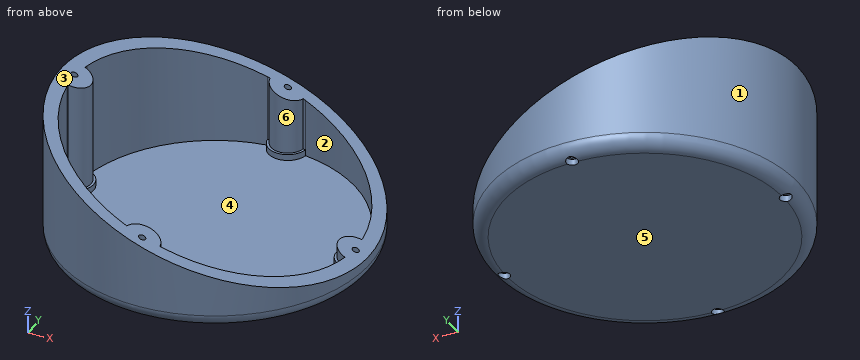
from build123d import *

# Parameters (mm, degrees)
SKETCH_1_R                = 57
EXTRUDE_1_DEPTH           = 50
CUT_EXTRUDE_1_DEPTH       = 95.857788294
CUT_EXTRUDE_1_DEPTH_BACK  = 95.857788294
FILLET_1_R                = 5
HOLE_WIZARD_1_D           = 2.4
HOLE_WIZARD_1_CBORE_D     = 4.3
HOLE_WIZARD_1_CBORE_DEPTH = 2.3
PATTERN_CIRCULAR_1_COUNT  = 4
SHELL_START               = 5
SHELL_1_DEPTH             = 43.047767655
SHELL_START_2             = 7.3
SHELL_1_2_DEPTH           = 40.747767655


# Read off the part's stored shape, not the designer's step: 抽壳1
with BuildPart() as part:
    # 草图1 → 凸台-拉伸1 (new body)
    with BuildSketch(Plane.XY):
        Circle(SKETCH_1_R)
    extrude(amount=EXTRUDE_1_DEPTH)

    # 草图2 → 切除-拉伸1 (cut, two sides: drawn at the far end of the back side and taken through both)
    with BuildSketch(Plane(origin=(0, 0, 0), x_dir=(1, 0, 0), z_dir=(0, 1, 0)).offset(-CUT_EXTRUDE_1_DEPTH_BACK)):
        Polygon((-57, -50), (57, -50), (57, -8.507393294), align=None)
    extrude(amount=CUT_EXTRUDE_1_DEPTH + CUT_EXTRUDE_1_DEPTH_BACK, mode=Mode.SUBTRACT)

    # 圆角1
    fillet_1_edges = [part.edges().sort_by_distance(p)[0] for p in [
        (-57, 0, 0),
    ]]
    fillet(fillet_1_edges, radius=FILLET_1_R)

    # 打孔尺寸(%根据)内六角圆柱头螺钉的类型1 (through all)
    with Locations(Plane(origin=(0, 0, 0), x_dir=(-1, 0, 0), z_dir=(0, 0, -1))):
        with Locations((0, 52.5)):
            hole_wizard_1 = CounterBoreHole(HOLE_WIZARD_1_D / 2, HOLE_WIZARD_1_CBORE_D / 2, HOLE_WIZARD_1_CBORE_DEPTH)

    # 阵列(圆周)1: 打孔尺寸(%根据)内六角圆柱头螺钉的类型1 ×4 about axis
    pattern_circular_1_axis = Axis((0, 0, 0), (0, 0, 1))
    for i in range(1, PATTERN_CIRCULAR_1_COUNT):
        add(hole_wizard_1.rotate(pattern_circular_1_axis, i * 360 / PATTERN_CIRCULAR_1_COUNT), mode=Mode.SUBTRACT)

    # 抽壳1 outline → 抽壳1 (cut)
    with BuildSketch(Plane.XY.offset(SHELL_START)):
        with BuildLine():
            ThreePointArc((7.081896621, -51.5155), (36.769552622, -36.769552622), (51.5155, -7.081896621))
            ThreePointArc((51.5155, -7.081896621), (45.35, 0), (51.5155, 7.081896621))
            ThreePointArc((51.5155, 7.081896621), (36.769552622, 36.769552622), (7.081896621, 51.5155))
            ThreePointArc((7.081896621, 51.5155), (0, 45.35), (-7.081896621, 51.5155))
            ThreePointArc((-7.081896621, 51.5155), (-36.769552622, 36.769552622), (-51.5155, 7.081896621))
            ThreePointArc((-51.5155, 7.081896621), (-45.35, 0), (-51.5155, -7.081896621))
            ThreePointArc((-51.5155, -7.081896621), (-36.769552622, -36.769552622), (-7.081896621, -51.5155))
            ThreePointArc((-7.081896621, -51.5155), (0, -45.35), (7.081896621, -51.5155))
        make_face()
    extrude(amount=SHELL_1_DEPTH, mode=Mode.SUBTRACT)

    # Shell 1 2 outline → Shell 1 2 (cut)
    with BuildSketch(Plane.XY.offset(SHELL_START_2)):
        with BuildLine():
            ThreePointArc((51.5155, 7.081896621), (45.35, 0), (51.5155, -7.081896621))
            ThreePointArc((51.5155, -7.081896621), (51.57804505, -6.610996049), (51.636285714, -6.139543764))
            ThreePointArc((51.636285714, -6.139543764), (46.3, 0), (51.636285714, 6.139543764))
            ThreePointArc((51.636285714, 6.139543764), (51.57804505, 6.610996049), (51.5155, 7.081896621))
        make_face()
        with BuildLine():
            ThreePointArc((6.139543764, -51.636285714), (6.610996049, -51.57804505), (7.081896621, -51.5155))
            ThreePointArc((7.081896621, -51.5155), (0, -45.35), (-7.081896621, -51.5155))
            ThreePointArc((-7.081896621, -51.5155), (-6.610996049, -51.57804505), (-6.139543764, -51.636285714))
            ThreePointArc((-6.139543764, -51.636285714), (0, -46.3), (6.139543764, -51.636285714))
        make_face()
        with BuildLine():
            ThreePointArc((-7.081896621, 51.5155), (0, 45.35), (7.081896621, 51.5155))
            ThreePointArc((7.081896621, 51.5155), (6.610996049, 51.57804505), (6.139543764, 51.636285714))
            ThreePointArc((6.139543764, 51.636285714), (0, 46.3), (-6.139543764, 51.636285714))
            ThreePointArc((-6.139543764, 51.636285714), (-6.610996049, 51.57804505), (-7.081896621, 51.5155))
        make_face()
        with BuildLine():
            ThreePointArc((-51.636285714, -6.139543764), (-51.57804505, -6.610996049), (-51.5155, -7.081896621))
            ThreePointArc((-51.5155, -7.081896621), (-45.35, 0), (-51.5155, 7.081896621))
            ThreePointArc((-51.5155, 7.081896621), (-51.57804505, 6.610996049), (-51.636285714, 6.139543764))
            ThreePointArc((-51.636285714, 6.139543764), (-46.3, 0), (-51.636285714, -6.139543764))
        make_face()
    extrude(amount=SHELL_1_2_DEPTH, mode=Mode.SUBTRACT)


solid = part.part
The listing builds one solid part. Answer for the finished solid, in the listing's coordinates (mm). Face numbers are marked on the shaded views. A direction names the side the tool comes from. Give positions to 0.01 mm unless a question says otherwise; leave off trailing zeros. Write each loop counter-clockwise with the first axis right and the second up, starting at its lowest first coordinate (ties: lowest second). Pieces come first, ordered by that corner, then holes. Notation, with made-up numbers: (82, 8) - (108, 8) arc R32 cw to (108, 46) - close; hole circle Ø6 at (-1, 67). An arc over 180 degrees is marked (long way). One line per question, with ' | ' between items. Start each with the question number.
1. Determine the mould class of the marked faces 1, 2, 3 and 4 for opening direction Y: +Y half, -Y half, draft (parallel to the pull), parting line (faces both ways), or undercut.
2. Straight lines are drawn through the part: line 1 (Y direction, x = 0, z = 1); line 2 (Y direction, x = 0, z = 20); line 3 (X direction, y = 0, z = 27). For each, find the intervals that lie inside material, in ascending order.
3. For the marked faces 5 and 6, determine the directions among +Z, -Z, +X, -X, +Y, -Y from which every point of the face is accessible in a straight line to the end or side of a thin tool.
4. Section A-A, the plane z = 19 is taken. Determine the outline of the cut face in (x, y), then the cut area to 3 significant figures.
5. Section B-B, the plane z = 45 is taken. Determine the outline of the cut face in (x, y).
6. Given P1, Ø1, axis at y = 11.5, z = 42.5, coming from the +X side; P2, Ø2, axis at x = -53.5, y = -1, coming from the -Z side; P3, Ø3.5, axis at x = 0, y = -52.5, coming from the +Z side, each flat-ended and moving along its own axis, determine where each tip first touches the part or whether it passes through.
Result:
1) face 1: parting line | face 2: undercut | face 3: draft | face 4: undercut
2) line 1: y = -55 to -54.65, -50.35 to 50.35, 54.65 to 55 | line 2: y = -57 to -53.7, -51.3 to -46.3, 46.3 to 51.3, 53.7 to 57 | line 3: x = -57 to -53.7, -51.3 to -46.3
3) face 5: -Z, +X, -X, +Y, -Y | face 6: +Z
4) outline: (-51.64, -6.14) arc R6.2 ccw to (-51.64, 6.14) arc R52 cw to (-51.52, 7.08) arc R52 cw to (-7.08, 51.52) arc R52 cw to (-6.14, 51.64) arc R6.2 ccw to (6.14, 51.64) arc R52 cw to (7.08, 51.52) arc R52 cw to (28.17, 43.71) - (28.17, 49.55) arc R57 ccw (long way) to (28.17, -49.55) - (28.17, -43.71) arc R52 cw to (7.08, -51.52) arc R52 cw to (6.14, -51.64) arc R6.2 ccw to (-6.14, -51.64) arc R52 cw to (-7.08, -51.52) arc R52 cw to (-51.52, -7.08) arc R52 cw to start; hole circle Ø2.4 at (-52.5, 0); hole circle Ø2.4 at (0, -52.5); hole circle Ø2.4 at (0, 52.5) | area: 1,300 mm2
5) outline: (-51.64, -6.14) arc R6.2 ccw to (-51.64, 6.14) arc R52 cw to (-51.52, 7.08) arc R52 cw to (-43.26, 28.85) - (-43.26, 37.11) arc R57 ccw to (-43.26, -37.11) - (-43.26, -28.85) arc R52 cw to (-51.52, -7.08) arc R52 cw to start; hole circle Ø2.4 at (-52.5, 0)
6) P1: stops at x = -50.6 | P2: stops at z = 0.19 | P3: stops at z = 29.89
